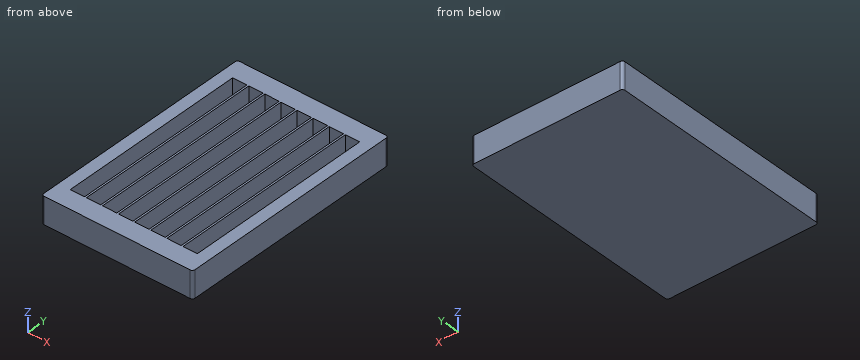
from build123d import *

# Parameters (mm, degrees)
SKIZZE1_W                       = 10
SKIZZE1_H                       = 54
AUFSATZ_LINEAR_AUSTRAGEN1_DEPTH = 15
SCHALE1_T                       = -1
LINEARES_MUSTER1_COUNT          = 8
LINEARES_MUSTER1_PITCH          = 9
SKIZZE2_W                       = 84.48
SKIZZE2_H                       = 127.76
SKIZZE2_W_2                     = 73
SKIZZE2_H_2                     = 108
AUFSATZ_LINEAR_AUSTRAGEN2_DEPTH = 15
VERRUNDUNG1_R                   = 1.5


with BuildPart() as part:
    # Skizze1 → Aufsatz-Linear austragen1 (new body)
    with BuildSketch(Plane.XY):
        with Locations((-5, 27)):
            Rectangle(SKIZZE1_W, SKIZZE1_H)
    extrude(amount=AUFSATZ_LINEAR_AUSTRAGEN1_DEPTH)

    # Schale1
    schale1_openings = [part.faces().sort_by_distance(p)[0] for p in [
        (-5, 27, 15),
        (-5, 0, 7.5),
    ]]
    offset(amount=SCHALE1_T, openings=schale1_openings, kind=Kind.INTERSECTION)


with BuildPart() as lineares_muster1_1:
    # Lineares Muster1: pattern copy
    add(part.part.moved(Location(Vector(-1, 0, 0) * (1 * LINEARES_MUSTER1_PITCH))))


with BuildPart() as lineares_muster1_2:
    # Lineares Muster1: pattern copy
    add(part.part.moved(Location(Vector(-1, 0, 0) * (2 * LINEARES_MUSTER1_PITCH))))


with BuildPart() as lineares_muster1_3:
    # Lineares Muster1: pattern copy
    add(part.part.moved(Location(Vector(-1, 0, 0) * (3 * LINEARES_MUSTER1_PITCH))))


with BuildPart() as lineares_muster1_4:
    # Lineares Muster1: pattern copy
    add(part.part.moved(Location(Vector(-1, 0, 0) * (4 * LINEARES_MUSTER1_PITCH))))


with BuildPart() as lineares_muster1_5:
    # Lineares Muster1: pattern copy
    add(part.part.moved(Location(Vector(-1, 0, 0) * (5 * LINEARES_MUSTER1_PITCH))))


with BuildPart() as lineares_muster1_6:
    # Lineares Muster1: pattern copy
    add(part.part.moved(Location(Vector(-1, 0, 0) * (6 * LINEARES_MUSTER1_PITCH))))


with BuildPart() as lineares_muster1_7:
    # Lineares Muster1: pattern copy
    add(part.part.moved(Location(Vector(-1, 0, 0) * (7 * LINEARES_MUSTER1_PITCH))))


with BuildPart() as part_1:
    add(part.part)

    # Kombinieren1: read off the stored shape, not the designer's step
    # Kombinieren1: union Lineares Muster1_1, Lineares Muster1_2, Lineares Muster1_3, Lineares Muster1_4, Lineares Muster1_5, Lineares Muster1_6, Lineares Muster1_7
    add(lineares_muster1_1.part)
    add(lineares_muster1_2.part)
    add(lineares_muster1_3.part)
    add(lineares_muster1_4.part)
    add(lineares_muster1_5.part)
    add(lineares_muster1_6.part)
    add(lineares_muster1_7.part)

    # Spiegeln1: part across plane


with BuildPart() as part_2:
    add(part_1.part)
    add(part_1.part.mirror(Plane(origin=(-63, 0, 15), x_dir=(0, 0, 1), z_dir=(0, 1, 0))))

    # Skizze2 → Aufsatz-Linear austragen2 (add)
    with BuildSketch(Plane.XY.offset(15)):
        with Locations((-36.5, 0)):
            Rectangle(SKIZZE2_W, SKIZZE2_H)
        with Locations((-36.5, 0)):
            Rectangle(SKIZZE2_W_2, SKIZZE2_H_2, mode=Mode.SUBTRACT)
    extrude(amount=-AUFSATZ_LINEAR_AUSTRAGEN2_DEPTH)

    # Verrundung1
    verrundung1_edges = [part_2.edges().sort_by_distance(p)[0] for p in [
        (-78.74, 63.88, 7.5),
        (-78.74, -63.88, 7.5),
        (5.74, -63.88, 7.5),
        (5.74, 63.88, 7.5),
    ]]
    fillet(verrundung1_edges, radius=VERRUNDUNG1_R)


solid = part_2.part
For this review, take the finished solid that the model builds, in its own axes (mm). Round coordinates to 2 decimals unless told otherwise and drop trailing zeros. Write each loop counter-clockwise with the first axis right and the second up, starting at its lowest first coordinate (ties: lowest second). Pieces come first, ordered by that corner, then holes. Notation, with made-up numbers: M 28,-26.5 L 64,-26.5 A20 cw 64,-22.5 Z; hole C 75.25,8 d8. An arc over 180 degrees is marked long. Write item = value, one per line. Start each with the question number.
(1) We need section B-B (z = 8.5). Give the number of separate pieces and of enclosed holes in the cut face, then the cut area to 3 significant figures.
(2) For line 1 along Y through (x, z) = (-38.5, 4); line 2 along Z through (x, y) = (-61, -6), list the stretches that pass through material, from the lowest coordinate up.
(3) We need section A-A (x = -32.5). Give the boundary of the cut face in (y, z).
(4) Clearance check with flat-ended pins moving along their axes: pin 1 Ø12 at (x, y) = (-65.5, 9) entering from +Z; pin 2 Ø2 at (x, y) = (-14.5, 45) entering from +Z. State where each tip first meets the part, or that it passes through.
Results found:
q1.separate_pieces = 1
q1.enclosed_holes = 8
q1.area = 4,010 mm²
q2.line_1 = -63.88 to -53, 53 to 63.88
q2.line_2 = 0 to 1
q3.outline = M -63.88,0 L 63.88,0 L 63.88,15 L 53,15 L 53,1 L -53,1 L -53,15 L -63.88,15 Z
q4.pin_1 = 15
q4.pin_2 = 1
